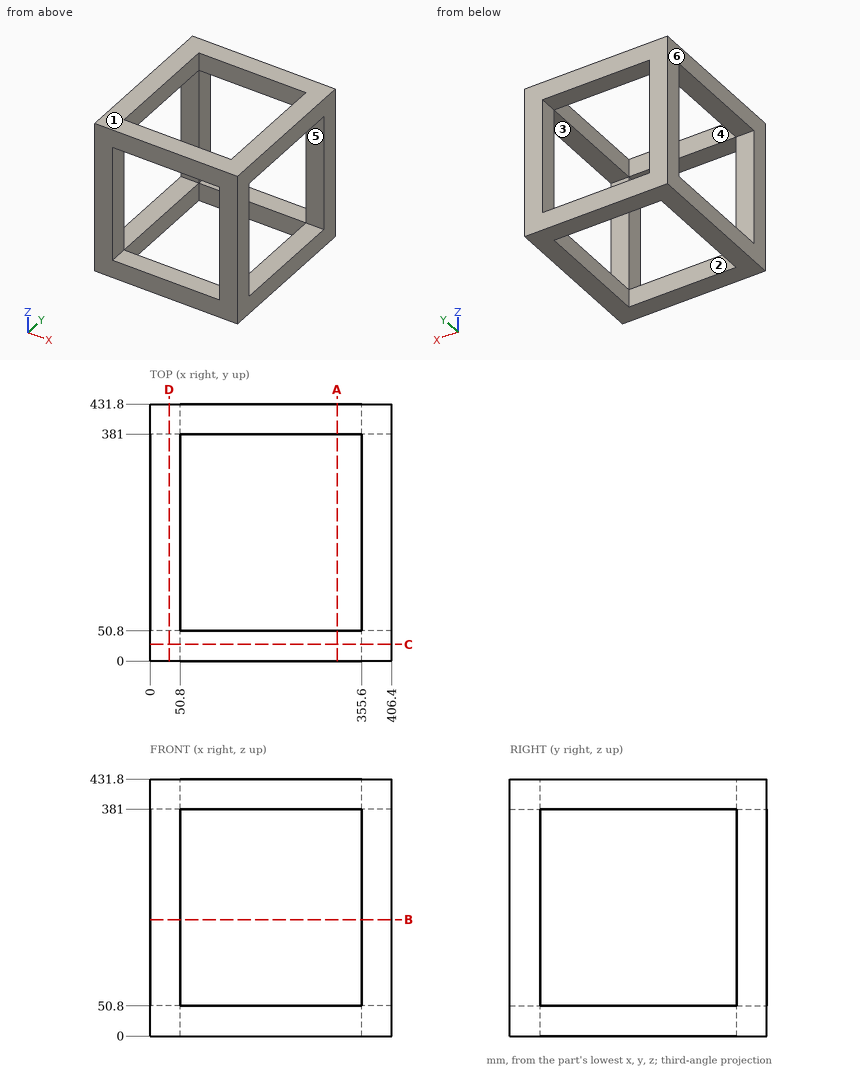
Design review of the part shown in the three views and the two pictorial views. Dimensions are in mm from the part's minimum x, y and z. A direction names the side the tool comes from. Coordinates: 2 decimals unless noted, no trailing zeros. Order: outer loops, then holes, each group sorted by start corner. A loop starts at its lowest first (then second) coordinate and runs counter-clockwise, first axis right, second up.
1) Wall thickness on line 1 along Z through (x, y) = (293, 32); line 2 along X through (y, z) = (245, 29): over which ranges is each line inside the solid? List them lowest first.
2) For the marked faces 1, 2 and 3, list the 3-axis set-ups (+Z, -Z, +X, -X, +Y, -Y) from which the entire face can be reached by the end or side of a thin tool; tool diameter is ignored.
3) Take a section at B-B, the plane z = 195.5. Give the boundary of the cut face in (x, y), and give its area (3 significant figures).
4) Take a section at A-A, the plane x = 314.5. Give the boundary of the cut face in (y, z), and give its area (3 significant figures).
5) Take a section at D-D, the plane x = 32. Give the boundary of the cut face in (y, z), and give its area (3 significant figures).
6) Mouldability with a two-part tool opening along X and no side actions: class the marked faces 4, 5 and 6 as +X half, -X half, draft (parallel to the pull), parting line (faces both ways), or undercut.
7) Clearance check with a flat-ended pin moving along its axis: pin 1 (15 mm diameter, centred on x = 387, y = 163, fed in from -Z). State where the tip first meets the part, or that it passes through.
8) Take a section at C-C, the plane y = 28. Give the boundary of the cut face in (x, z).
Returned:
1. line 1: z = 0 to 50.8, 381 to 431.8
1. line 2: x = 0 to 50.8, 355.6 to 406.4
2. face 1: +Z, +X, -X, +Y, -Y
2. face 2: +Z, -Z
2. face 3: +X, -X
3. outline: (0, 0) - (50.8, 0) - (50.8, 50.8) - (0, 50.8) - close; (0, 381) - (50.8, 381) - (50.8, 431.8) - (0, 431.8) - close; (355.6, 0) - (406.4, 0) - (406.4, 50.8) - (355.6, 50.8) - close; (355.6, 381) - (406.4, 381) - (406.4, 431.8) - (355.6, 431.8) - close
3. area: 10,300 mm2
4. outline: (0, 0) - (50.8, 0) - (50.8, 50.8) - (0, 50.8) - close; (0, 381) - (50.8, 381) - (50.8, 431.8) - (0, 431.8) - close; (381, 0) - (431.8, 0) - (431.8, 50.8) - (381, 50.8) - close; (381, 381) - (431.8, 381) - (431.8, 431.8) - (381, 431.8) - close
4. area: 10,300 mm2
5. outline: (0, 0) - (431.8, 0) - (431.8, 431.8) - (0, 431.8) - close; hole (50.8, 50.8) - (381, 50.8) - (381, 381) - (50.8, 381) - close
5. area: 77,400 mm2
6. face 4: undercut
6. face 5: draft
6. face 6: -X half
7. pin 1: stops at z = 0
8. outline: (0, 0) - (406.4, 0) - (406.4, 431.8) - (0, 431.8) - close; hole (50.8, 50.8) - (355.6, 50.8) - (355.6, 381) - (50.8, 381) - close
